Work out the finished part from the listing and answer in its coordinate system (mm). Give positions to 0.01 mm unless a question says otherwise; leave off trailing zeros. Loops run counter-clockwise (first coordinate to the right, second up) from the corner with the lowest first, then second, coordinate; pieces in that order, holes last. Notation, with made-up numbers: (31.5, 79.25) - (68.5, 79.25) arc R23 cw to (68.5, 115.25) - close; hole circle Ø5 at (21.5, 0). An arc over 180 degrees is marked (long way). Use CSV: the item, a comma, the result in double quotes.
from build123d import *

# Parameters (mm, degrees)
F0_W      = 72.1
F0_H      = 144.9
F0_W_2    = 65.9861192107
F0_H_2    = 121.5704865754
F1_DEPTH  = 6.4
F2_R      = 3
F3_R      = 1.6199699766
F3_R_2    = 1.0969181454
F3_W      = 6.3781980425
F3_H      = 0.7731094956
F3_W_2    = 4.1554919444
F3_H_2    = 1.0630339384
F4_DEPTH  = 0.1
F6_D      = 0.28
F13_D     = 2
F13_DEPTH = 0.5
F13_TIP   = 0.600860619


# Not quite as in the source:
# - the program builds the solid bodies; features that only make, move or delete a surface that nothing else refers to are left out


with BuildPart() as f1:
    # F0 (on Front) → F1 (new body)
    with BuildSketch(Plane.XZ):
        with Locations((21.9475186944, 24.6742434323)):
            Rectangle(F0_W, F0_H)
        with Locations((21.9411961734, 23.4142001718)):
            Rectangle(F0_W_2, F0_H_2, mode=Mode.SUBTRACT)
    extrude(amount=F1_DEPTH)

    # F2
    f2_edges = [f1.edges().sort_by_distance(p)[0] for p in [
        (21.947519, -6.4, 97.124243),
        (-14.102481, -6.4, 24.674243),
        (21.947519, -6.4, -47.775757),
        (57.997519, -6.4, 24.674243),
    ]]
    fillet(f2_edges, radius=F2_R)

    # F3 (on face) → F4 (join, symmetric)
    with BuildSketch(Plane.XZ.offset(6.4)):
        with Locations((37.9579253495, 88.9658480883)):
            Circle(F3_R)
        with Locations((37.9579253495, 88.9658480883)):
            Circle(F3_R_2, mode=Mode.SUBTRACT)
        with Locations((27.0376754925, 89.3524028361)):
            Rectangle(F3_W, F3_H)
        with Locations((4.2791056912, 89.4973650575)):
            Rectangle(F3_W_2, F3_H_2)
    extrude(amount=F4_DEPTH, both=True)

    # F6 (through all)
    with Locations(Plane.YZ.offset(57.9975186944)):
        with Locations((-1.4492898481, -30.8446902782), (-1.4492898481, 0.1785024215)):
            Hole(F6_D / 2)

    # F13
    with Locations(Plane.XZ.offset(6.4)):
        with Locations((37.9579253495, 88.9658480883)):
            Hole(F13_D / 2, depth=F13_DEPTH)
            with Locations((0, 0, -(F13_DEPTH + F13_TIP / 2))):  # 118° drill point
                Cone(0, F13_D / 2, F13_TIP, mode=Mode.SUBTRACT)


solid = f1.part
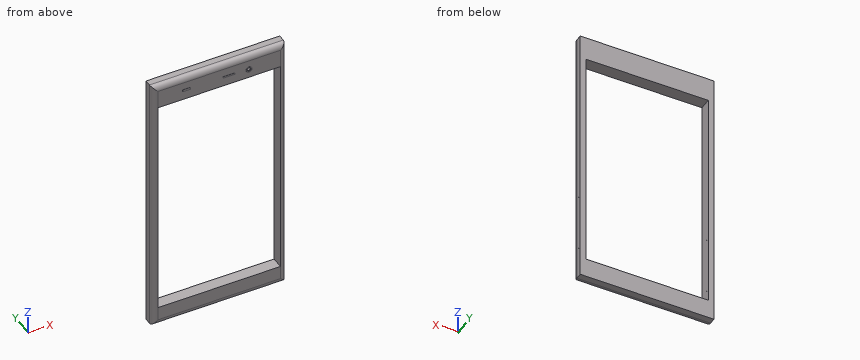
Item 1: Find the intervals of material crossed by line 1 (X direction, y = -2.25, z = 48.5); line 2 (Z direction, x = 0.5, y = -3); line 3 (X direction, y = -5.75, z = 63.5), in increasing order.
Determined:
line 1,"x = -14.1 to -11.05, 54.93 to 58"
line 2,"z = -47.78 to -37.37, 84.2 to 97.12"
line 3,"x = -12.97 to -11.05, 54.93 to 56.86"
Item 2: A cutting plane is placed at B-B on z = 24.5. Determine the outline of the cut face in (x, y).
Determined:
outline,"(-14.1, -3.4) arc R3 ccw to (-11.1, -6.4) - (-11.05, -6.4) - (-11.05, 0) - (-14.1, 0) - close; (54.93, -6.4) - (55, -6.4) arc R3 ccw to (58, -3.4) - (58, 0) - (54.93, 0) - close"
Item 3: Given P1, Ø1.5, axis at y = -5.5, z = 79, coming from the -X side, flat-ended and moving along its own axis, determine where the tip first touches the part or whether it passes through.
Determined:
P1,"stops at x = -13.78"
Item 4: A cutting plane is placed at C-C on x = 17. Determine the outline of the cut face in (y, z), and give its area (3 significant figures).
Determined:
outline,"(-6.4, -44.78) arc R3 ccw to (-3.4, -47.78) - (0, -47.78) - (0, -37.37) - (-6.4, -37.37) - close; (-6.4, 84.2) - (0, 84.2) - (0, 97.12) - (-3.4, 97.12) arc R3 ccw to (-6.4, 94.12) - close"
area,"145 mm²"
Item 5: A cutting plane is placed at A-A on x = 27.5. Determine the outline of the cut face in (y, z).
Determined:
outline,"(-6.5, 88.97) - (-6.4, 88.97) - (-6.4, 84.2) - (0, 84.2) - (0, 97.12) - (-3.4, 97.12) arc R3 ccw to (-6.4, 94.12) - (-6.4, 89.74) - (-6.5, 89.74) - close; (-6.4, -44.78) arc R3 ccw to (-3.4, -47.78) - (0, -47.78) - (0, -37.37) - (-6.4, -37.37) - close"
